from build123d import *

# Parameters (mm, degrees)
SKETCH1_W                = 47
SKETCH1_H                = 10
BOSS_EXTRUDE1_DEPTH      = 10
BOSS_EXTRUDE3_DEPTH      = 15
BOSS_EXTRUDE3_DEPTH_BACK = 15
SKETCH5_W                = 8.120903277
SKETCH5_H                = 37.25
CUT_EXTRUDE1_DEPTH       = 57.27735446


with BuildPart() as part:
    # Sketch1 → Boss-Extrude1 (new body)
    with BuildSketch(Plane.XY):
        with Locations((23.5, 5)):
            Rectangle(SKETCH1_W, SKETCH1_H)
    extrude(amount=BOSS_EXTRUDE1_DEPTH)

    # Sketch5 → Boss-Extrude3 (add, two sides: drawn at the far end of the back side and taken through both)
    with BuildSketch(Plane.XY.offset(5).offset(-BOSS_EXTRUDE3_DEPTH_BACK)):
        with Locations((42.939548362, 5)):
            Rectangle(SKETCH5_W, SKETCH5_H)
    extrude(amount=BOSS_EXTRUDE3_DEPTH + BOSS_EXTRUDE3_DEPTH_BACK)

    # Sketch6 → Cut-Extrude1 (cut, through all)
    with BuildSketch(Plane.XY.offset(10)):
        Polygon((0, 10), (2.679491924, 10), (0, 0), align=None)
    extrude(amount=-CUT_EXTRUDE1_DEPTH, mode=Mode.SUBTRACT)


solid = part.part
Verification items for the finished model (mm, model axes). A direction names the side the tool comes from. Give positions to 0.01 mm unless a question says otherwise; leave off trailing zeros. Loops run counter-clockwise (first coordinate to the right, second up) from the corner with the lowest first, then second, coordinate; pieces in that order, holes last. Notation, with made-up numbers: (44.5, 72) - (60.5, 72) arc R13 cw to (60.5, 95) - close; hole circle Ø10 at (0.25, 29.25). An arc over 180 degrees is marked (long way). Write each question's results on one line, items separated by ' | '.
1) Depth check by flat-ended pin: P1, Ø8, axis at x = 20, z = 5, coming from the +Y side; P2, Ø5, axis at x = 14.5, z = 4.5, coming from the -Y side; P3, Ø11, axis at x = 26.5, y = 6, coming from the +Z side. Enter the tip coordinate at first touch or a pass-through.
Solution:
P1: y = 10 | P2: y = 0 | P3: z = 10
2) Sectioned sample at A-A on z = 7.75. Record the boundary of the cut face in (x, y) (1 decimal), plus the area to 3 significant figures.
Solution:
outline: (0, 0) - (38.9, 0) - (38.9, -13.6) - (47, -13.6) - (47, 23.6) - (38.9, 23.6) - (38.9, 10) - (2.7, 10) - close | area: 678 mm2
3) Tool access check on faces 1 (the flat face through (19, 5, 0)), 2 (the flat face through (19, 0, 5)), 3 (the flat face through (43, 5, -10)), 4 (the flat face through (19, 5, 10)), 5 (the flat face through (21, 10, 5)). Record the directions out of +Z, -Z, +X, -X, +Y, -Y that give a thin tool (end or side, any length) a straight path to the whole face; none if there is none.
Solution:
face 1: -Z, -X, +Y, -Y | face 2: +Z, -Z, -X, -Y | face 3: -Z, +X, -X, +Y, -Y | face 4: +Z, -X, +Y, -Y | face 5: +Z, -Z, -X, +Y
4) Material ranges on L1, parallel to Z at x = 12.5, y = 1; L2, parallel to X at y = 3, z = -7.75, recorded low to high. Write a range as from..to.
Solution:
L1: 0..10 | L2: 38.88..47
5) Sectioned sample at B-B on x = 20. Record the boundary of the cut face in (y, z), plus the area to 3 significant figures.
Solution:
outline: (0, 0) - (10, 0) - (10, 10) - (0, 10) - close | area: 100 mm2
6) Sectioned sample at C-C on y = -2. Record the boundary of the cut face in (x, z).
Solution:
outline: (38.88, -10) - (47, -10) - (47, 20) - (38.88, 20) - close
7) Sectioned sample at D-D on y = 8.5. Record the boundary of the cut face in (x, z), plus the area to 3 significant figures.
Solution:
outline: (2.28, 0) - (38.88, 0) - (38.88, -10) - (47, -10) - (47, 20) - (38.88, 20) - (38.88, 10) - (2.28, 10) - close | area: 610 mm2
